Input: part model. Units: mm. Frame: model coordinates. Give positions to 0.01 mm unless a question says otherwise; leave off trailing zeros. Write each loop counter-clockwise with the first axis right and the second up, starting at its lowest first coordinate (ties: lowest second). Pieces come first, ordered by that corner, then holes.
Autodesk Inventor part; units mm, degrees
ref_plane "YZ Plane" through (0, 0, 0) normal (1, 0, 0) x (0, 1, 0)
ref_plane "XZ Plane" through (0, 0, 0) normal (0, 1, 0) x (-1, 0, 0)
ref_plane "XY Plane" through (0, 0, 0) normal (0, 0, 1) x (1, 0, 0)
sketch "Sketch1" plane through (0, 0, 0) normal (0, 0, 1) x (1, 0, 0)
  line L0 (-30, -30) -> (30, -30)
  line L1 (30, -30) -> (30, 30)
  line L2 (30, 30) -> (-30, 30)
  line L3 (-30, 30) -> (-30, -30)
  line L4 (-30, -30) -> (30, 30) construction
  line L5 (30, -30) -> (-30, 30) construction
  circle A0 centre (0, 0) radius 29
  circle A1 centre (-25, 25) radius 2
  circle A2 centre (25, 25) radius 2
  circle A3 centre (25, -25) radius 2
  circle A4 centre (-25, -25) radius 2
  line L6 (-25, 25) -> (25, 25) construction
  line L7 (25, 25) -> (25, -25) construction
  line L8 (25, -25) -> (-25, -25) construction
  dimension "d0" = 60
  dimension "d3" = 50
  dimension "d4" = 4
  dimension "d5" = 58
extrude "Extrusion1" add sketch "Sketch1" along normal blind 15.3
fillet "Fillet1" radius 3.175 4 edges at (30, 30, 7.65) (30, -30, 7.65) (-30, 30, 7.65) (-30, -30, 7.65)
properties part number "Fan"
Q1. Mould query, pull axis X, two halves, no side actions, for faces 1 (the cylindrical face through (23.4, 26.2, 7.5)), 2 (the cylindrical face through (29.09, 29.05, 7.76)), 3 (the flat face through (-30, 0, 8)), 4 (the flat face through (0, 30, 8)). Classes: +X half, -X half, draft (parallel to the pull), parting line (faces both ways), or undercut.
Q2. Pin query (flat end, axial travel): pin 1 (4.5 mm diameter, centred on x = 25, y = -25, fed in from +Z); pin 2 (3.5 mm diameter, centred on x = -25, y = -25, fed in from +Z). Return the tip coordinate at first contact, or that it passes through.
Q3. Section A-A, the plane x = 0. Return the cut outline in (y, z), then the cut area to 3 significant figures.
Q4. Section D-D, the plane x = -25. Return the cut outline in (y, z).
Q5. Section B-B, the plane z = 4.75. Return the cut outline in (x, y) (3 decimals), then the cut area to 3 significant figures.
Q6. Section C-C, the plane y = -12.5. Return the cut outline in (x, z), then the cut area to 3 significant figures.
Q7. Material intervals for line 1 along Y through (x, z) = (25, 5); line 2 along Y through (x, z) = (-11, 12); line 3 along Y through (x, z) = (2.5, 5.5), sorted ascending.
Solutions:
1. face 1: undercut
1. face 2: +X half
1. face 3: -X half
1. face 4: draft
2. pin 1: stops at z = 15.3
2. pin 2: passes through
3. outline: (-30, 0) - (-29, 0) - (-29, 15.3) - (-30, 15.3) - close; (29, 0) - (30, 0) - (30, 15.3) - (29, 15.3) - close
3. area: 30.6 mm2
4. outline: (-30, 0) - (-27, 0) - (-27, 15.3) - (-30, 15.3) - close; (-23, 0) - (-14.7, 0) - (-14.7, 15.3) - (-23, 15.3) - close; (14.7, 0) - (23, 0) - (23, 15.3) - (14.7, 15.3) - close; (27, 0) - (30, 0) - (30, 15.3) - (27, 15.3) - close
5. outline: (-30, -26.825) arc R3.175 ccw to (-26.825, -30) - (26.825, -30) arc R3.175 ccw to (30, -26.825) - (30, 26.825) arc R3.175 ccw to (26.825, 30) - (-26.825, 30) arc R3.175 ccw to (-30, 26.825) - close; hole circle Ø58 at (0, 0); hole circle Ø4 at (-25, -25); hole circle Ø4 at (-25, 25); hole circle Ø4 at (25, -25); hole circle Ø4 at (25, 25)
5. area: 899 mm2
6. outline: (-30, 0) - (-26.17, 0) - (-26.17, 15.3) - (-30, 15.3) - close; (26.17, 0) - (30, 0) - (30, 15.3) - (26.17, 15.3) - close
6. area: 117 mm2
7. line 1: y = -30 to -27, -23 to -14.7, 14.7 to 23, 27 to 30
7. line 2: y = -30 to -26.83, 26.83 to 30
7. line 3: y = -30 to -28.89, 28.89 to 30
